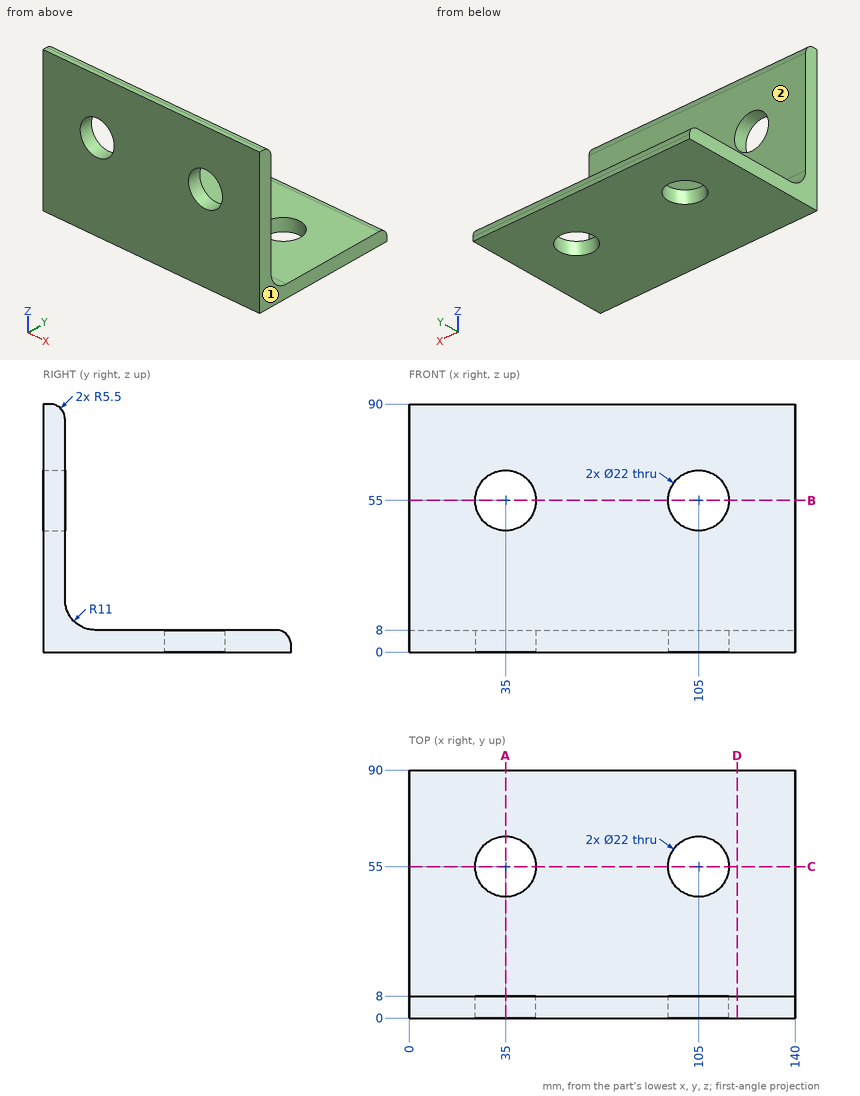
Geometry: see drawing. Coordinates: mm, zero at the bounding-box minimum. A direction names the side the tool comes from. Round coordinates to 2 decimals unless told otherwise and drop trailing zeros. Loops run counter-clockwise (first coordinate to the right, second up) from the corner with the lowest first, then second, coordinate; pieces in that order, holes last. Notation, with made-up numbers: (46, 2.25) - (105, 2.25) arc R29 cw to (105, 34.25) - close; hole circle Ø2 at (3, 71). An arc over 180 degrees is marked (long way). One line per item, written item: value. Start each with the question number.
(1) Section D-D, the plane x = 119. Return loops of the section in (y, z).
(2) Section A-A, the plane x = 35. Return loops of the section in (y, z), plus the area to 3 significant figures.
(3) Access query for the marked faces 1 and 2. Directions: +Z, -Z, +X, -X, +Y, -Y. A direction counts if a zero-diameter tool reaches every point of the face in a straight line with its end or side. Return the directions, or none.
(4) Section B-B, the plane z = 55. Return loops of the section in (x, y).
(5) Ray query, line 1 (X direction, y = 55, z = 2); line 2 (Z direction, x = 105, y = 2.75); line 3 (Y direction, x = 35.5, z = 24). Return the intervals inside material, ascending. Write a range as [from, to].
(6) Contact query for flat-ended pins moving along their axis: P1, Ø5, axis at x = 24, y = 22, coming from the +Z side; P2, Ø2, axis at x = 119, z = 34, coming from the +Y side. Output: stop coordinate, or through.
Results below:
1. outline: (0, 0) - (90, 0) - (90, 2.5) arc R5.5 ccw to (84.5, 8) - (19, 8) arc R11 cw to (8, 19) - (8, 84.5) arc R5.5 ccw to (2.5, 90) - (0, 90) - close
2. outline: (0, 0) - (44, 0) - (44, 8) - (19, 8) arc R11 cw to (8, 19) - (8, 44) - (0, 44) - close; (0, 66) - (8, 66) - (8, 84.5) arc R5.5 ccw to (2.5, 90) - (0, 90) - close; (66, 0) - (90, 0) - (90, 2.5) arc R5.5 ccw to (84.5, 8) - (66, 8) - close
2. area: 1,040 mm^2
3. face 1: +Z, -Z, +X, +Y, -Y
3. face 2: +Z, +X, -X, +Y
4. outline: (0, 0) - (24, 0) - (24, 8) - (0, 8) - close; (46, 0) - (94, 0) - (94, 8) - (46, 8) - close; (116, 0) - (140, 0) - (140, 8) - (116, 8) - close
5. line 1: [0, 24], [46, 94], [116, 140]
5. line 2: [0, 44], [66, 89.99]
5. line 3: [0, 8]
6. P1: z = 8
6. P2: y = 8
